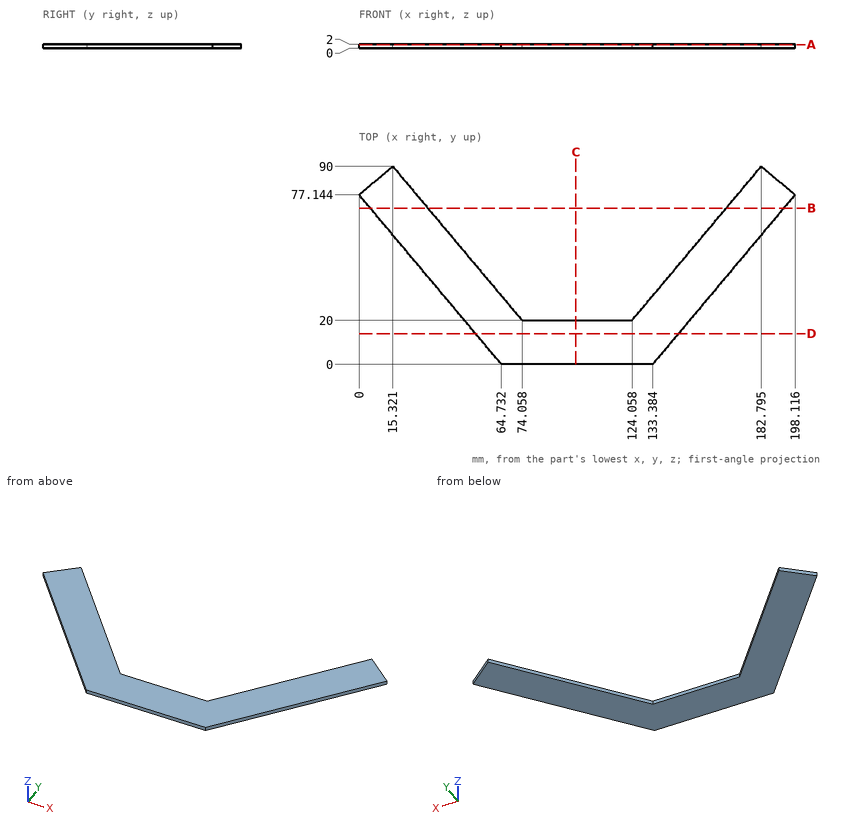
Drawing for the job (mm, zero at the part's lowest x, y, z). Give positions to 0.01 mm unless a question says otherwise; leave off trailing zeros. Loops run counter-clockwise (first coordinate to the right, second up) from the corner with the lowest first, then second, coordinate; pieces in that order, holes last.
1) Probe line 1 along X through (y, z) = (48, 0.8) (1 decimal); line 2 along X through (y, z) = (53.5, 0.8) (1 decimal); line 3 along Y through (x, z) = (77, 0.55). List the from-to ranges inside material, lowest first.
Values follow:
line 1: x = 24.5 to 50.6, 147.6 to 173.7
line 2: x = 19.8 to 45.9, 152.2 to 178.3
line 3: y = 0 to 20
2) Band-saw the part on A-A on z = 1.7. List the corners of the cut face in (x, y) (1 decimal).
Values follow:
outline: (0, 77.1) - (64.7, 0) - (133.4, 0) - (198.1, 77.1) - (182.8, 90) - (124.1, 20) - (74.1, 20) - (15.3, 90) - close
3) Band-saw the part on C-C on x = 98.5. List the corners of the cut face in (y, z).
Values follow:
outline: (0, 0) - (20, 0) - (20, 2) - (0, 2) - close
4) Band-saw the part on D-D on y = 14. List the corners of the cut face in (x, z).
Values follow:
outline: (52.98, 0) - (145.13, 0) - (145.13, 2) - (52.98, 2) - close
5) Band-saw the part on B-B on y = 71. List the corners of the cut face in (x, z) (1 decimal).
Values follow:
outline: (5.2, 0) - (31.3, 0) - (31.3, 2) - (5.2, 2) - close; (166.9, 0) - (193, 0) - (193, 2) - (166.9, 2) - close
